Geometry: final body of the model. Coordinates: model frame, mm. A direction names the side the tool comes from. Coordinates: 2 decimals unless noted, no trailing zeros. Write each loop counter-clockwise with the first axis right and the second up, starting at its lowest first coordinate (ties: lowest second). Pieces come first, ordered by that corner, then holes.
from build123d import *

# Parameters (mm, degrees)
SKETCH_1_R               = 15
EXTRUDE_1_DEPTH          = 2
SKETCH_1_7_R             = 2.5
EXTRUDE_2_DEPTH          = 10
SKETCH_2_R               = 0.35
CUT_EXTRUDE_1_DEPTH      = 4
CUT_EXTRUDE_3_DEPTH      = 24.452078799
CUT_EXTRUDE_3_DEPTH_BACK = 24.452078799
SKETCH_3_R               = 1


with BuildPart() as part:
    # Sketch 1 → Extrude 1 (new body)
    with BuildSketch(Plane(origin=(0, 0, 0), x_dir=(1, 0, 0), z_dir=(0, 1, 0))):
        with Locations(Location((0, 0, 0), (0, 0, 270))):
            Circle(SKETCH_1_R)
    extrude(amount=EXTRUDE_1_DEPTH)

    # Sketch 1_7 → Extrude 2 (add)
    with BuildSketch(Plane(origin=(0, 0, 0), x_dir=(1, 0, 0), z_dir=(0, 1, 0))):
        with Locations(Location((0, 0, 0), (0, 0, 270))):
            Circle(SKETCH_1_7_R)
    extrude(amount=EXTRUDE_2_DEPTH)

    # Sketch 2 → Cut-Extrude 1 (cut)
    with BuildSketch(Plane(origin=(0, 10, 0), x_dir=(1, 0, 0), z_dir=(0, 1, 0))):
        with Locations(Location((0, 0, 0), (0, 0, 270))):
            Circle(SKETCH_2_R)
    extrude(amount=-CUT_EXTRUDE_1_DEPTH, mode=Mode.SUBTRACT)

    # Sketch 3 → Cut-Extrude 3 (cut, two sides: drawn at the far end of the back side and taken through both)
    with BuildSketch(Plane.XY.offset(-CUT_EXTRUDE_3_DEPTH_BACK)):
        with Locations(Location((0, 6, 0), (0, 0, 89.999999999))):
            Circle(SKETCH_3_R)
    extrude(amount=CUT_EXTRUDE_3_DEPTH + CUT_EXTRUDE_3_DEPTH_BACK, mode=Mode.SUBTRACT)


solid = part.part
Item 1: Section A-A, the plane z = 0. Output: boundary loops of the cut face in (x, y), plus the area to 3 significant figures.
Derived:
outline: (-15, 0) - (15, 0) - (15, 2) - (2.5, 2) - (2.5, 10) - (0.35, 10) - (0.35, 6.94) arc R1 cw (long way) to (-0.35, 6.94) - (-0.35, 10) - (-2.5, 10) - (-2.5, 2) - (-15, 2) - close
area: 94.7 mm2
Item 2: Pull-direction query (X, two-part tool) for faces 1 (the cylindrical face through (0.6, 5.2, 0)), 2 (the cylindrical face through (0.66, 0.986, -14.985)), 3 (the flat face through (0, 10, 1)); classes: released by +X, released by -X, zero draft, split by the parting line, or undercut.
Derived:
face 1: undercut
face 2: split by the parting line
face 3: zero draft
Item 3: Section B-B, the plane x = 0. Output: boundary loops of the cut face in (y, z).
Derived:
outline: (0, -15) - (2, -15) - (2, -2.5) - (5, -2.5) - (5, 2.5) - (2, 2.5) - (2, 15) - (0, 15) - close; (7, -2.5) - (10, -2.5) - (10, -0.35) - (7, -0.35) - close; (7, 0.35) - (10, 0.35) - (10, 2.5) - (7, 2.5) - close
Item 4: Set-up query: faces 4 (the flat face through (0, 0, 0)), 5 (the cylindrical face through (-2.22, 5.94, 1.15)). Return all of +Z, -Z, +X, -X, +Y, -Y with unobstructed straight access to the full face (end or side cutting, diameter ignored); none if empty.
Derived:
face 4: +Z, -Z, +X, -X, -Y
face 5: +Y
Item 5: Pin query (flat end, axial travel): pin 1 (6 mm diameter, centred on x = -2.5, y = 2, fed in from -Z); pin 2 (2.5 mm diameter, centred on x = 0, y = 6, fed in from -Z); pin 3 (6 mm diameter, centred on x = 9.5, z = 4.5, fed in from +Y). Return the tip coordinate at first contact, or that it passes through.
Derived:
pin 1: stops at z = -15
pin 2: stops at z = -2.5
pin 3: stops at y = 2
Item 6: Section C-C, the plane y = 7.5. Output: boundary loops of the cut face in (x, z).
Derived:
outline: circle Ø5 at (0, 0); hole circle Ø0.7 at (0, 0)
Item 7: Material intervals for probe 1 along X at (y, z) = (8.2, 0); probe 2 along Y at (x, z) = (13.25, -1); probe 3 along X at (y, z) = (6, -0.05), sorted ascending.
Derived:
probe 1: x = -2.5 to -0.35, 0.35 to 2.5
probe 2: y = 0 to 2
probe 3: x = -2.5 to -1, 1 to 2.5
Item 8: Section D-D, the plane y = 1.25. Output: boundary loops of the cut face in (x, z).
Derived:
outline: circle Ø30 at (0, 0)
